from build123d import *

# Parameters (mm, degrees)
SKETCH1_W               = 55.88
SKETCH1_H               = 69.85
BOSS_EXTRUDE1_DEPTH     = 185.928
CAVITY2_DEPTH           = 55.88
CUT_EXTRUDE1_DEPTH      = 207.326968872
CUT_EXTRUDE1_DEPTH_BACK = 207.326968872
CAVITY3_START           = 155.611951918
CAVITY3_OUTLINE_W       = 55.88
CAVITY3_OUTLINE_H       = 16.002
CAVITY3_DEPTH           = 13.861518057
CAVITY3_START_2         = 43.09882965
CAVITY3_2_OUTLINE_W     = 55.88
CAVITY3_2_OUTLINE_H     = 16.002
CAVITY3_2_DEPTH         = 6.77134799
CAVITY3_START_3         = 103.490840018
CAVITY3_3_OUTLINE_W     = 55.88
CAVITY3_3_OUTLINE_H     = 16.002
CAVITY3_3_DEPTH         = 5.588
CUT_EXTRUDE2_DEPTH      = 207.326968872
CUT_EXTRUDE2_DEPTH_BACK = 207.326968872
SKETCH4_W               = 12.644530025
SKETCH4_H               = 16.002
SKETCH4_W_2             = 38.9131119
SKETCH4_W_3             = 46.000662378
SKETCH4_W_4             = 39.28882965
FILLET1_R               = 7.62


# Read off the part's stored shape, not the designer's step: Cavity2, Cavity3
with BuildPart() as part:
    # Sketch1 → Boss-Extrude1 (new body)
    with BuildSketch(Plane.XY):
        with Locations((27.94, 34.925)):
            Rectangle(SKETCH1_W, SKETCH1_H)
    extrude(amount=BOSS_EXTRUDE1_DEPTH)

    # Cavity2 outline → Cavity2 (cut)
    with BuildSketch(Plane.YZ):
        with BuildLine():
            Line((0, 185.372681959), (0, 178.347013566))
            ThreePointArc((0, 178.347013566), (0.234915375, 179.528012907), (0.903897763, 180.529215804))
            Line((0.903897763, 180.529215804), (5.797646215, 185.422964256))
            ThreePointArc((5.797646215, 185.422964256), (7.204232738, 185.702751711), (8.001, 184.510305235))
            Line((8.001, 184.510305235), (8.001, 181.3052))
            ThreePointArc((8.001, 181.3052), (8.506885168, 180.083885168), (9.7282, 179.578))
            Line((9.7282, 179.578), (10.3378, 179.578))
            ThreePointArc((10.3378, 179.578), (11.559114832, 180.083885168), (12.065, 181.3052))
            Line((12.065, 181.3052), (12.065, 182.478305235))
            ThreePointArc((12.065, 182.478305235), (11.049, 183.494305235), (12.065, 184.510305235))
            Line((12.065, 184.510305235), (12.065, 185.928))
            Line((12.065, 185.928), (0.555318041, 185.928))
            Line((0.555318041, 185.928), (0, 185.372681959))
        make_face()
        with BuildLine():
            Line((0, 160.528), (0, 156.668018354))
            ThreePointArc((0, 156.668018354), (1.097837867, 157.474813069), (2.011305235, 156.464))
            Line((2.011305235, 156.464), (6.738477062, 156.464))
            ThreePointArc((6.738477062, 156.464), (7.643464695, 157.473916954), (8.74621772, 156.684695417))
            ThreePointArc((8.74621772, 156.684695417), (10.673815789, 157.855184211), (11.844304583, 159.78278228))
            ThreePointArc((11.844304583, 159.78278228), (11.055083046, 160.885535305), (12.065, 161.790522938))
            Line((12.065, 161.790522938), (12.065, 166.517694765))
            ThreePointArc((12.065, 166.517694765), (11.049, 167.533694765), (12.065, 168.549694765))
            Line((12.065, 168.549694765), (12.065, 169.7228))
            ThreePointArc((12.065, 169.7228), (11.559114832, 170.944114832), (10.3378, 171.45))
            Line((10.3378, 171.45), (9.7282, 171.45))
            ThreePointArc((9.7282, 171.45), (8.506885168, 170.944114832), (8.001, 169.7228))
            Line((8.001, 169.7228), (8.001, 166.517694765))
            ThreePointArc((8.001, 166.517694765), (7.204232738, 165.325248289), (5.797646215, 165.605035744))
            Line((5.797646215, 165.605035744), (0.903897763, 170.498784196))
            ThreePointArc((0.903897763, 170.498784196), (0.234915375, 171.499987093), (0, 172.680986434))
            Line((0, 172.680986434), (0, 165.655318041))
            Line((0, 165.655318041), (2.923964256, 162.731353785))
            ThreePointArc((2.923964256, 162.731353785), (3.203751711, 161.324767262), (2.011305235, 160.528))
            Line((2.011305235, 160.528), (0, 160.528))
        make_face()
        with BuildLine():
            Line((0, 20.272681959), (0, 13.247013566))
            ThreePointArc((0, 13.247013566), (0.234915375, 14.428012907), (0.903897763, 15.429215804))
            Line((0.903897763, 15.429215804), (5.797646215, 20.322964256))
            ThreePointArc((5.797646215, 20.322964256), (7.204232738, 20.602751711), (8.001, 19.410305235))
            Line((8.001, 19.410305235), (8.001, 16.2052))
            ThreePointArc((8.001, 16.2052), (8.506885168, 14.983885168), (9.7282, 14.478))
            Line((9.7282, 14.478), (10.3378, 14.478))
            ThreePointArc((10.3378, 14.478), (11.559114832, 14.983885168), (12.065, 16.2052))
            Line((12.065, 16.2052), (12.065, 17.378305235))
            ThreePointArc((12.065, 17.378305235), (11.049, 18.394305235), (12.065, 19.410305235))
            Line((12.065, 19.410305235), (12.065, 24.137477062))
            ThreePointArc((12.065, 24.137477062), (11.055083046, 25.042464695), (11.844304583, 26.14521772))
            ThreePointArc((11.844304583, 26.14521772), (10.673815789, 28.072815789), (8.74621772, 29.243304583))
            ThreePointArc((8.74621772, 29.243304583), (7.643464695, 28.454083046), (6.738477062, 29.464))
            Line((6.738477062, 29.464), (2.011305235, 29.464))
            ThreePointArc((2.011305235, 29.464), (1.097837867, 28.453186931), (0, 29.259981646))
            Line((0, 29.259981646), (0, 25.4))
            Line((0, 25.4), (2.011305235, 25.4))
            ThreePointArc((2.011305235, 25.4), (3.203751711, 24.603232738), (2.923964256, 23.196646215))
            Line((2.923964256, 23.196646215), (0, 20.272681959))
        make_face()
        with BuildLine():
            Line((12.065, 0), (12.065, 1.417694765))
            ThreePointArc((12.065, 1.417694765), (11.049, 2.433694765), (12.065, 3.449694765))
            Line((12.065, 3.449694765), (12.065, 4.6228))
            ThreePointArc((12.065, 4.6228), (11.559114832, 5.844114832), (10.3378, 6.35))
            Line((10.3378, 6.35), (9.7282, 6.35))
            ThreePointArc((9.7282, 6.35), (8.506885168, 5.844114832), (8.001, 4.6228))
            Line((8.001, 4.6228), (8.001, 1.417694765))
            ThreePointArc((8.001, 1.417694765), (7.204232738, 0.225248289), (5.797646215, 0.505035744))
            Line((5.797646215, 0.505035744), (0.903897763, 5.398784196))
            ThreePointArc((0.903897763, 5.398784196), (0.234915375, 6.399987093), (0, 7.580986434))
            Line((0, 7.580986434), (0, 0.555318041))
            Line((0, 0.555318041), (0.555318041, 0))
            Line((0.555318041, 0), (12.065, 0))
        make_face()
    extrude(amount=CAVITY2_DEPTH, mode=Mode.SUBTRACT)

    # Sketch2 → Cut-Extrude1 (cut, two sides: drawn at the far end of the back side and taken through both)
    with BuildSketch(Plane(origin=(55.88, 0, 0), x_dir=(0, 0, -1), z_dir=(1, 0, 0)).offset(-CUT_EXTRUDE1_DEPTH_BACK)):
        Polygon((-185.928, 53.848), (-185.928, 12.065), (-187.786827766, 0), (-183.387405269, 0), (-186.368592882, 6.922214935), (-185.928, 7.695543501), (-179.578, 10.033), (-179.578, 53.848), align=None)
        Polygon((-171.45, 36.068), (-171.45, 10.033), (-163.181232022, 10.033), (-165.655318041, 0), (-20.272681959, 0), (-21.714355158, 8.498769389), (-14.478, 10.033), (-14.478, 36.068), align=None)
        Polygon((0.982362905, -0.670371441), (0, 12.065), (0, 53.848), (-6.35, 53.848), (-6.35, 10.033), (-1.572527278, 10.022034637), (0.234962195, 6.712117206), (-3.38001675, -0.670371441), align=None)
    extrude(amount=CUT_EXTRUDE1_DEPTH + CUT_EXTRUDE1_DEPTH_BACK, mode=Mode.SUBTRACT)

    # Cavity3 outline → Cavity3 (cut)
    with BuildSketch(Plane.XY.offset(CAVITY3_START)):
        with Locations((27.94, 61.849)):
            Rectangle(CAVITY3_OUTLINE_W, CAVITY3_OUTLINE_H)
    extrude(amount=CAVITY3_DEPTH, mode=Mode.SUBTRACT)

    # Cavity3 2 outline → Cavity3 2 (cut)
    with BuildSketch(Plane.XY.offset(CAVITY3_START_2)):
        with Locations((27.94, 61.849)):
            Rectangle(CAVITY3_2_OUTLINE_W, CAVITY3_2_OUTLINE_H)
    extrude(amount=CAVITY3_2_DEPTH, mode=Mode.SUBTRACT)

    # Cavity3 3 outline → Cavity3 3 (cut)
    with BuildSketch(Plane.XY.offset(CAVITY3_START_3)):
        with Locations((27.94, 61.849)):
            Rectangle(CAVITY3_3_OUTLINE_W, CAVITY3_3_OUTLINE_H)
    extrude(amount=CAVITY3_3_DEPTH, mode=Mode.SUBTRACT)

    # Sketch4 → Cut-Extrude2 (cut, two sides: drawn at the far end of the back side and taken through both)
    with BuildSketch(Plane(origin=(55.88, 0, 0), x_dir=(0, 0, -1), z_dir=(1, 0, 0)).offset(-CUT_EXTRUDE2_DEPTH_BACK)):
        with Locations((-179.605734987, 61.849)):
            Rectangle(SKETCH4_W, SKETCH4_H)
        with Locations((-132.345395968, 61.849)):
            Rectangle(SKETCH4_W_2, SKETCH4_H)
        with Locations((-76.680508829, 61.849)):
            Rectangle(SKETCH4_W_3, SKETCH4_H)
        with Locations((-19.644414825, 61.849)):
            Rectangle(SKETCH4_W_4, SKETCH4_H)
    extrude(amount=CUT_EXTRUDE2_DEPTH + CUT_EXTRUDE2_DEPTH_BACK, mode=Mode.SUBTRACT)

    # Fillet1
    fillet1_edges = [part.edges().sort_by_distance(p)[0] for p in [
        (27.94, 36.068, 14.478),
        (27.94, 36.068, 171.45),
    ]]
    fillet(fillet1_edges, radius=FILLET1_R)


solid = part.part
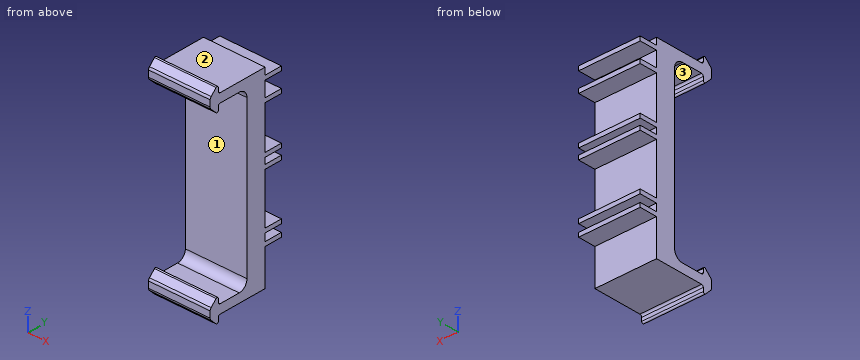
The model under review builds one solid part; all positions refer to its coordinate system, in mm. Face numbers are marked on the shaded views. A direction names the side the tool comes from. Round coordinates to 2 decimals unless told otherwise and drop trailing zeros. Order: outer loops, then holes, each group sorted by start corner. A loop starts at its lowest first (then second) coordinate and runs counter-clockwise, first axis right, second up. Notation, with made-up numbers: (17.25, -23) -> (42.25, -23) arc R11 cw to (42.25, -13) -> close; hole circle Ø11 at (7.25, -29). An arc over 180 degrees is marked (long way). Use CSV: the item, a comma, the result in double quotes. Start each with the question number.
(1) Consider section A-A on y = 23. Write out the cut boundary in (x, z), and give its area (3 significant figures).
(2) Consider section B-B on z = 136.5. Write out the cut boundary in (x, y).
(3) Wall thickness on probe 1 along Z at (x, y) = (51.5, 60); probe 2 along Z at (x, y) = (33.5, 25); probe 3 along Z at (x, y) = (25, 39.5): over which ranges is each line inside the solid? List them lowest first. Write a range as from..to.
(4) Insertion check: pin 1 (16.5 mm diameter, centred on x = 24.5, z = 30, fed in from +Y); pin 2 (10 mm diameter, centred on y = 62.5, z = 93.5, fed in from -X); pin 3 (5 mm diameter, centred on x = 31.5, y = 64.5, fed in from -Z); pin 4 (2 mm diameter, centred on x = 23, y = 34.5, fed in from -Z). Each pin has a flat end and moves straight along its axis. Give the tip position at first contact, or say it passes through.
(5) Tool access review of the marked faces 1, 2 and 3: name each direction out of +Z, -Z, +X, -X, +Y, -Y from which nothing blocks a thin tool from reaching the whole face with its end or side.
Responses:
1,outline,"(0, 6.35) -> (55.88, 6.35) -> (55.88, 14.48) -> (0, 14.48) -> close; (0, 171.45) -> (55.88, 171.45) -> (55.88, 179.58) -> (0, 179.58) -> close"
1,area,"908 mm²"
2,outline,"(0, 36.07) -> (55.88, 36.07) -> (55.88, 53.85) -> (0, 53.85) -> close"
3,probe 1,"39.29..43.1, 49.87..53.68, 99.68..103.49, 109.08..112.89, 151.8..155.61, 169.47..173.28"
3,probe 2,"6.35..14.48, 171.45..179.58"
3,probe 3,"6.35..179.58"
4,pin 1,"y = 53.85"
4,pin 2,"through"
4,pin 3,"z = 39.29"
4,pin 4,"z = 6.35"
5,face 1,"+X, -X, -Y"
5,face 2,"+Z, +X, -X, +Y"
5,face 3,"+X, -X"
